```python
from build123d import *

# Parameters (mm, degrees)
SKETCH1_R           = 2.6
BOSS_EXTRUDE1_DEPTH = 3
SKETCH2_R           = 3.5
BOSS_EXTRUDE2_DEPTH = 4
CUT_EXTRUDE1_DEPTH  = 3
SKETCH4_R           = 1.4
CUT_EXTRUDE2_DEPTH  = 111.335850928


with BuildPart() as part:
    # Sketch1 → Boss-Extrude1 (new body)
    with BuildSketch(Plane.XY):
        with BuildLine():
            Line((3, 0), (70, 0))
            Line((70, 0), (82, 0))
            ThreePointArc((82, 0), (84.121320344, 0.878679656), (85, 3))
            Line((85, 3), (85, 9))
            ThreePointArc((85, 9), (84.121320344, 11.121320344), (82, 12))
            Line((82, 12), (73, 12))
            ThreePointArc((73, 12), (70.878679656, 12.878679656), (70, 15))
            Line((70, 15), (70, 55))
            ThreePointArc((70, 55), (70.878679656, 57.121320344), (73, 58))
            Line((73, 58), (82, 58))
            ThreePointArc((82, 58), (84.121320344, 58.878679656), (85, 61))
            Line((85, 61), (85, 67))
            ThreePointArc((85, 67), (84.121320344, 69.121320344), (82, 70))
            Line((82, 70), (67, 70))
            Line((67, 70), (3, 70))
            ThreePointArc((3, 70), (0.878679656, 69.121320344), (0, 67))
            Line((0, 67), (0, 3))
            ThreePointArc((0, 3), (0.878679656, 0.878679656), (3, 0))
        make_face()
        with Locations((79, 64)):
            Circle(SKETCH1_R, mode=Mode.SUBTRACT)
        with Locations((79, 6)):
            Circle(SKETCH1_R, mode=Mode.SUBTRACT)
    extrude(amount=BOSS_EXTRUDE1_DEPTH)

    # Sketch2 → Boss-Extrude2 (add)
    with BuildSketch(Plane.XY.offset(3)):
        with Locations(Location((5, 65, 0), (0, 0, 180))):
            Circle(SKETCH2_R)
        with Locations(Location((65, 65, 0), (0, 0, 180))):
            Circle(SKETCH2_R)
        with Locations(Location((65, 5, 0), (0, 0, 180))):
            Circle(SKETCH2_R)
        with Locations(Location((5, 5, 0), (0, 0, 180))):
            Circle(SKETCH2_R)
    extrude(amount=BOSS_EXTRUDE2_DEPTH)

    # Sketch3 → Cut-Extrude1 (cut)
    with BuildSketch(Plane.XY.offset(3)):
        Polygon((14, 60), (56, 60), (35, 39), align=None)
        Polygon((60, 56), (60, 14), (39, 35), align=None)
        Polygon((56, 10), (14, 10), (35, 31), align=None)
        Polygon((10, 14), (10, 56), (31, 35), align=None)
    extrude(amount=-CUT_EXTRUDE1_DEPTH, mode=Mode.SUBTRACT)

    # Sketch4 → Cut-Extrude2 (cut, through all)
    with BuildSketch(Plane.XY.offset(7)):
        with Locations((5, 65)):
            Circle(SKETCH4_R)
        with Locations((65, 65)):
            Circle(SKETCH4_R)
        with Locations((65, 5)):
            Circle(SKETCH4_R)
        with Locations((5, 5)):
            Circle(SKETCH4_R)
    extrude(amount=-CUT_EXTRUDE2_DEPTH, mode=Mode.SUBTRACT)


solid = part.part
```
Could you check a few things on this model? Use its own coordinates, in mm. A direction names the side the tool comes from. Round coordinates to 2 decimals unless told otherwise and drop trailing zeros. Loops run counter-clockwise (first coordinate to the right, second up) from the corner with the lowest first, then second, coordinate; pieces in that order, holes last. Notation, with made-up numbers: M 3.5,7 L 39.5,7 A34 cw 39.5,42 Z; hole C 78.5,23.5 d3. An arc over 180 degrees is marked long. Put each result on its own line as item: value.
Q1. Imagine slicing it at D-D (y = 37). Write out the boundary of the cut face in (x, z), then the cut area to 3 significant figures.
Check result:
outline: M 0,0 L 10,0 L 10,3 L 0,3 Z; M 29,0 L 41,0 L 41,3 L 29,3 Z; M 60,0 L 70,0 L 70,3 L 60,3 Z
area: 96.0 mm2
Q2. Thinking about a two-plate mould opening in X: for faces 5 (the face through (85, 6, 1)), 6 (the face through (63, 65, 7)), 7 (the face through (45, 21, 2)), which applies, released by +X, released by -X, zero draft, split by the parting line, or undercut?
Check result:
face 5: released by +X
face 6: zero draft
face 7: undercut
Q3. Imagine slicing it at A-A (y = 49). Write out the boundary of the cut face in (x, z), then the cut area to 3 significant figures.
Check result:
outline: M 0,0 L 10,0 L 10,3 L 0,3 Z; M 17,0 L 25,0 L 25,3 L 17,3 Z; M 45,0 L 53,0 L 53,3 L 45,3 Z; M 60,0 L 70,0 L 70,3 L 60,3 Z
area: 108 mm2
Q4. Imagine slicing it at C-C (x = 65). Write out the boundary of the cut face in (y, z), then the cut area to 3 significant figures.
Check result:
outline: M 0,0 L 3.6,0 L 3.6,7 L 1.5,7 L 1.5,3 L 0,3 Z; M 6.4,0 L 63.6,0 L 63.6,7 L 61.5,7 L 61.5,3 L 8.5,3 L 8.5,7 L 6.4,7 Z; M 66.4,0 L 70,0 L 70,3 L 68.5,3 L 68.5,7 L 66.4,7 Z
area: 227 mm2
Q5. Imagine slicing it at B-B (z = 6). Write out the boundary of the cut face in (x, y), then the cut area to 3 significant figures.
Check result:
outline: C 5,5 d7; C 5,65 d7; C 65,5 d7; C 65,65 d7; hole C 5,5 d2.8; hole C 5,65 d2.8; hole C 65,5 d2.8; hole C 65,65 d2.8
area: 129 mm2
Q6. On a 3-axis mill with a long thin cutter (end or side, diameter ignored), from which of +Z, -Z, +X, -X, +Y, -Y can I reach the whole of each face in a straight line? I mean faces 1 (the face through (21, 25, 2)), 2 (the face through (84.1, 58.86, 1.48)), 3 (the face through (43, 70, 1)), 4 (the face through (1.767, 6.341, 4.972)). Say none if no direction works.
Check result:
face 1: +Z, -Z
face 2: +Z, -Z, +X
face 3: +Z, -Z, +X, -X, +Y
face 4: +Z
Q7. For pin 1 (3.5 mm diameter, centred on y = 27, z = 1, fed in from +X); pin 2 (12 mm diameter, centred on x = 41, y = 25, fed in from +Z), each with a flat end and sliding along its axis, tell me the tip position at first contact or that it passes through.
Check result:
pin 1: x = 70
pin 2: z = 3
Q8. I need wall thicknesses on probe 1 along Y at (x, z) = (35, 2); probe 2 along Y at (x, z) = (32, 2); probe 3 along Y at (x, z) = (25, 1). Which ranges of each line are inside material? Lowest first, please.
Check result:
probe 1: 0 to 10, 31 to 39, 60 to 70
probe 2: 0 to 10, 28 to 42, 60 to 70
probe 3: 0 to 10, 21 to 29, 41 to 49, 60 to 70
